```python
from build123d import *

# Parameters (mm, degrees)
SKETCH1_R               = 28
SKETCH1_R_2             = 16
BOSS_EXTRUDE1_DEPTH     = 35
BOSS_EXTRUDE4_DEPTH     = 31
BOSS_EXTRUDE8_DEPTH     = 9
BOSS_EXTRUDE10_START    = 12
SKETCH6_8_R             = 25
SKETCH6_8_R_2           = 12.5
BOSS_EXTRUDE10_DEPTH    = 12
SKETCH6_9_R             = 25
SKETCH6_9_R_2           = 12.5
BOSS_EXTRUDE11_DEPTH    = 34
CUT_EXTRUDE2_DEPTH      = 143.246265329
CUT_EXTRUDE2_DEPTH_BACK = 143.246265329
SKETCH8_W               = 34
SKETCH8_H               = 56
SKETCH9_W               = 18
SKETCH9_H               = 36
BOSS_EXTRUDE12_DEPTH    = 55
CUT_EXTRUDE3_DEPTH      = 150.916643506
CUT_EXTRUDE3_DEPTH_BACK = 150.916643506
SKETCH12_R              = 12.5
SKETCH18_W              = 42
SKETCH18_H              = 36
BOSS_EXTRUDE15_DEPTH    = 30
CUT_EXTRUDE8_DEPTH      = 167.03011775
CUT_EXTRUDE8_DEPTH_BACK = 167.03011775
SKETCH30_R              = 7.5
SKETCH31_R              = 18
BOSS_EXTRUDE18_DEPTH    = 24
CUT_EXTRUDE9_DEPTH      = 176.926120858
CUT_EXTRUDE9_DEPTH_BACK = 176.926120858
SKETCH30_2_R            = 7.5


with BuildPart() as part:
    # Sketch1 → Boss-Extrude1 (new, symmetric)
    with BuildSketch(Plane(origin=(0, 0, 0), x_dir=(0, 0, -1), z_dir=(1, 0, 0))):
        Circle(SKETCH1_R)
        Circle(SKETCH1_R_2, mode=Mode.SUBTRACT)
    extrude(amount=BOSS_EXTRUDE1_DEPTH, both=True)

    # Sketch2 → Boss-Extrude4 (add, symmetric)
    with BuildSketch(Plane(origin=(0, 0, 0), x_dir=(0, 0, -1), z_dir=(1, 0, 0))):
        with BuildLine():
            Line((-25, 40), (25, 40))
            Line((25, 40), (25, 12.609520213))
            ThreePointArc((25, 12.609520213), (0, 28), (-25, 12.609520213))
            Line((-25, 12.609520213), (-25, 40))
        make_face()
    extrude(amount=BOSS_EXTRUDE4_DEPTH, both=True)

    # Sketch6 → Boss-Extrude8 (add, symmetric)
    with BuildSketch(Plane(origin=(0, 0, 0), x_dir=(0, 0, -1), z_dir=(1, 0, 0))):
        with BuildLine():
            Line((-25, 110), (-25, 40))
            Line((-25, 40), (25, 40))
            Line((25, 40), (25, 110))
            ThreePointArc((25, 110), (0, 85), (-25, 110))
        make_face()
    extrude(amount=BOSS_EXTRUDE8_DEPTH, both=True)

    # Sketch6_8 → Boss-Extrude10 (add)
    with BuildSketch(Plane(origin=(0, 0, 0), x_dir=(0, 0, -1), z_dir=(1, 0, 0)).offset(BOSS_EXTRUDE10_START)):
        with Locations((0, 110)):
            Circle(SKETCH6_8_R)
        with Locations((0, 110)):
            Circle(SKETCH6_8_R_2, mode=Mode.SUBTRACT)
    extrude(amount=-BOSS_EXTRUDE10_DEPTH)

    # Sketch6_9 → Boss-Extrude11 (add)
    with BuildSketch(Plane(origin=(0, 0, 0), x_dir=(0, 0, -1), z_dir=(1, 0, 0))):
        with Locations((0, 110)):
            Circle(SKETCH6_9_R)
        with Locations((0, 110)):
            Circle(SKETCH6_9_R_2, mode=Mode.SUBTRACT)
    extrude(amount=-BOSS_EXTRUDE11_DEPTH)

    # Sketch8 → Cut-Extrude2 (cut, two sides: drawn at the far end of the back side and taken through both)
    with BuildSketch(Plane.XY.offset(-CUT_EXTRUDE2_DEPTH_BACK)):
        Rectangle(SKETCH8_W, SKETCH8_H)
    extrude(amount=CUT_EXTRUDE2_DEPTH + CUT_EXTRUDE2_DEPTH_BACK, mode=Mode.SUBTRACT)

    # Sketch9 → Boss-Extrude12 (add)
    with BuildSketch(Plane.XY):
        with Locations((-11, 117)):
            Rectangle(SKETCH9_W, SKETCH9_H)
    extrude(amount=BOSS_EXTRUDE12_DEPTH)

    # Sketch12 → Cut-Extrude3 (cut, two sides: drawn at the far end of the back side and taken through both)
    with BuildSketch(Plane(origin=(0, 0, 0), x_dir=(0, 0, -1), z_dir=(1, 0, 0)).offset(-CUT_EXTRUDE3_DEPTH_BACK)):
        with Locations((0, 110)):
            Circle(SKETCH12_R)
    extrude(amount=CUT_EXTRUDE3_DEPTH + CUT_EXTRUDE3_DEPTH_BACK, mode=Mode.SUBTRACT)

    # Sketch18 → Boss-Extrude15 (add)
    with BuildSketch(Plane.XY.offset(55)):
        with Locations((-11, 117)):
            Rectangle(SKETCH18_W, SKETCH18_H)
    extrude(amount=BOSS_EXTRUDE15_DEPTH)

    # Sketch30 → Cut-Extrude8 (cut, two sides: drawn at the far end of the back side and taken through both)
    with BuildSketch(Plane.ZY.offset(11).offset(-CUT_EXTRUDE8_DEPTH_BACK)):
        with Locations((85, 117)):
            Circle(SKETCH30_R)
    extrude(amount=CUT_EXTRUDE8_DEPTH + CUT_EXTRUDE8_DEPTH_BACK, mode=Mode.SUBTRACT)

    # Sketch31 → Boss-Extrude18 (add, symmetric)
    with BuildSketch(Plane.ZY.offset(11)):
        with Locations((85, 117)):
            Circle(SKETCH31_R)
    extrude(amount=BOSS_EXTRUDE18_DEPTH, both=True)

    # Sketch30_2 → Cut-Extrude9 (cut, two sides: drawn at the far end of the back side and taken through both)
    with BuildSketch(Plane.ZY.offset(11).offset(-CUT_EXTRUDE9_DEPTH_BACK)):
        with Locations((85, 117)):
            Circle(SKETCH30_2_R)
    extrude(amount=CUT_EXTRUDE9_DEPTH + CUT_EXTRUDE9_DEPTH_BACK, mode=Mode.SUBTRACT)


solid = part.part
```
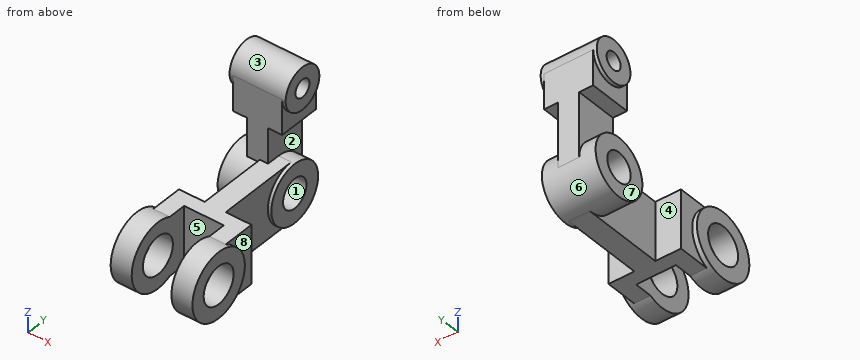
Source: CAD feature listing. Evaluate the final solid. Frame: model axes, mm. Face numbers are marked on the shaded views. A direction names the side the tool comes from. Coordinates: 2 decimals unless noted, no trailing zeros. Write each loop counter-clockwise with the first axis right and the second up, starting at its lowest first coordinate (ties: lowest second). Pieces come first, ordered by that corner, then holes. Notation, with made-up numbers: (39.5, -27.5) - (61.5, -27.5) arc R37 ccw to (61.5, 11.5) - close; hole circle Ø9 at (68.25, 65.5). An arc over 180 degrees is marked (long way). Answer as a JSON object with one key per item and string values.
Q1. Section query C-C, the plane y = 117. Output: boundary loops of the cut face in (x, z).
Ans:
{"outline": "(-35, 67) - (-32, 67) - (-32, 55) - (-20, 55) - (-20, 24) - (-34, 24) - (-34, 10.36) - (12, 10.36) - (12, 24) - (-2, 24) - (-2, 55) - (10, 55) - (10, 67) - (13, 67) - (13, 77.5) - (-35, 77.5) - close; (-35, 92.5) - (13, 92.5) - (13, 103) - (-35, 103) - close; (-34, -24) - (12, -24) - (12, -10.36) - (-34, -10.36) - close"}
Q2. Section query B-B, the plane z = 90. Output: boundary loops of the cut face in (x, y).
Ans:
{"outline": "(-35, 99.71) - (13, 99.71) - (13, 111.41) - (-35, 111.41) - close; (-35, 122.59) - (13, 122.59) - (13, 134.29) - (-35, 134.29) - close"}
Q3. Section query D-D, the plane x = 22.5. Output: boundary loops of the cut face in (y, z), plus the area to 3 significant figures.
Ans:
{"outline": "(12.61, -25) - (40, -25) - (40, 25) - (12.61, 25) arc R28 ccw (long way) to start; hole circle Ø32 at (0, 0)", "area": "2,480 mm2"}
Q4. Material intervals for line 1 (Y direction, x = -19, z = 0); line 2 (Y direction, x = -14, z = 85); line 3 (Z direction, x = 22, y = 0), sorted ascending. Write a range as [from, to].
Ans:
{"line 1": "y = [-28, -16], [16, 40], [85, 97.5], [122.5, 135]", "line 2": "y = [99, 109.5], [124.5, 135]", "line 3": "z = [-28, -16], [16, 28]"}
Q5. Draft query along Y for the marked faces 1, 2 and 3. Return one class per face: released by +Y, released by -Y, zero draft, split by the parting line, or undercut.
Ans:
{"face 1": "undercut", "face 2": "zero draft", "face 3": "split by the parting line"}
Q6. Set-up query: the marked faces 4, 5, 6, 7 and 8. Return all of +Z, -Z, +X, -X, +Y, -Y with unobstructed straight access to the full face (end or side cutting, diameter ignored); none if empty.
Ans:
{"face 4": "+Z, -Z, -X", "face 5": "+Z, -Z, -Y", "face 6": "none", "face 7": "-Z, -X, +Y", "face 8": "+X, +Y"}
Q7. First-contact query: pin 1 Ø3 at (x, y) = (-23, 8.5) entering from -Z; pin 2 Ø18 at (y, z) = (109, 78.5) entering from +X; pin 3 Ø25 at (y, z) = (114.5, -1.5) entering from -X. Flat tips, straight axial feed; report the tip coordinate or a pass-through.
Ans:
{"pin 1": "stops at z = -27.11", "pin 2": "stops at x = 13", "pin 3": "stops at x = -34"}
Q8. Section query A-A, the plane x = 4.5. Output: boundary loops of the cut face in (y, z), plus the area to 3 significant figures.
Ans:
{"outline": "(28, -25) - (110, -25) arc R25 ccw to (110, 25) - (28, 25) - close; (99, 55) - (135, 55) - (135, 85) arc R18 ccw to (99, 85) - close; hole circle Ø25 at (110, 0); hole circle Ø15 at (117, 85)", "area": "6,000 mm2"}
